from build123d import *

# Parameters (mm, degrees)
SKETCH1_W            = 85.6
SKETCH1_H            = 56
BOSS_EXTRUDE1_DEPTH  = 1.6
SKETCH2_W            = 21.3
SKETCH2_H            = 15.9
BOSS_EXTRUDE2_DEPTH  = 13.5
SKETCH3_W            = 17.4
SKETCH3_H            = 14.7
BOSS_EXTRUDE3_DEPTH  = 15.5
SKETCH4_W            = 16.8
SKETCH4_H            = 28.8
BOSS_EXTRUDE4_DEPTH  = 3.4
SKETCH5_W            = 24
SKETCH5_H            = 2.1
BOSS_EXTRUDE5_DEPTH  = 17.7
SKETCH6_W            = 10
SKETCH6_H            = 10
BOSS_EXTRUDE6_DEPTH  = 13.2
SKETCH7_R            = 4.15
BOSS_EXTRUDE7_DEPTH  = 9.5
SKETCH8_W            = 12
SKETCH8_H            = 11.5
BOSS_EXTRUDE8_DEPTH  = 10
SKETCH9_R            = 3.5
BOSS_EXTRUDE9_DEPTH  = 3.5
SKETCH10_W           = 33
SKETCH10_H           = 5.1
BOSS_EXTRUDE10_DEPTH = 8.3
SKETCH11_W           = 5.4
SKETCH11_H           = 7.5
BOSS_EXTRUDE11_DEPTH = 2.7
SKETCH12_W           = 15
SKETCH12_H           = 9
BOSS_EXTRUDE12_DEPTH = 6.2
SKETCH13_R           = 1.45
CUT_EXTRUDE1_DEPTH   = 6


with BuildPart() as part:
    # Sketch1 → Boss-Extrude1 (new body)
    with BuildSketch(Plane(origin=(0, 0, 0), x_dir=(1, 0, 0), z_dir=(0, 1, 0))):
        Rectangle(SKETCH1_W, SKETCH1_H)
    extrude(amount=BOSS_EXTRUDE1_DEPTH)

    # Sketch2 → Boss-Extrude2 (add)
    with BuildSketch(Plane(origin=(0, 1.6, 0), x_dir=(1, 0, 0), z_dir=(0, 1, 0))):
        with Locations((33.85, -18.45)):
            Rectangle(SKETCH2_W, SKETCH2_H)
    extrude(amount=BOSS_EXTRUDE2_DEPTH)

    # Sketch3 → Boss-Extrude3 (add)
    with BuildSketch(Plane(origin=(0, 1.6, 0), x_dir=(1, 0, 0), z_dir=(0, 1, 0))):
        with Locations((41.7, 2.65)):
            Rectangle(SKETCH3_W, SKETCH3_H)
    extrude(amount=BOSS_EXTRUDE3_DEPTH)

    # Sketch4 → Boss-Extrude4 (add)
    with BuildSketch(Plane.XZ):
        with Locations((-34.4, -1.5)):
            Rectangle(SKETCH4_W, SKETCH4_H)
    extrude(amount=BOSS_EXTRUDE4_DEPTH)

    # Sketch5 → Boss-Extrude5 (add)
    with BuildSketch(Plane.ZY.offset(42.8)):
        with Locations((-2.5, -1.65)):
            Rectangle(SKETCH5_W, SKETCH5_H)
    extrude(amount=BOSS_EXTRUDE5_DEPTH)

    # Sketch6 → Boss-Extrude6 (add)
    with BuildSketch(Plane(origin=(0, 1.6, 0), x_dir=(1, 0, 0), z_dir=(0, 1, 0))):
        with Locations((3.1, 23)):
            Rectangle(SKETCH6_W, SKETCH6_H)
    extrude(amount=BOSS_EXTRUDE6_DEPTH)

    # Sketch7 → Boss-Extrude7 (add)
    with BuildSketch(Plane(origin=(0, 0, -28), x_dir=(-1, 0, 0), z_dir=(0, 0, -1))):
        with Locations((-3.1, 9.4)):
            Circle(SKETCH7_R)
    extrude(amount=BOSS_EXTRUDE7_DEPTH)

    # Sketch8 → Boss-Extrude8 (add)
    with BuildSketch(Plane(origin=(0, 1.6, 0), x_dir=(1, 0, 0), z_dir=(0, 1, 0))):
        with Locations((22.5, 22.25)):
            Rectangle(SKETCH8_W, SKETCH8_H)
    extrude(amount=BOSS_EXTRUDE8_DEPTH)

    # Sketch9 → Boss-Extrude9 (add)
    with BuildSketch(Plane(origin=(0, 0, -28), x_dir=(-1, 0, 0), z_dir=(0, 0, -1))):
        with Locations((-22.5, 8.1)):
            Circle(SKETCH9_R)
    extrude(amount=BOSS_EXTRUDE9_DEPTH)

    # Sketch10 → Boss-Extrude10 (add)
    with BuildSketch(Plane(origin=(0, 1.6, 0), x_dir=(1, 0, 0), z_dir=(0, 1, 0))):
        with Locations((-25.6, 24.55)):
            Rectangle(SKETCH10_W, SKETCH10_H)
    extrude(amount=BOSS_EXTRUDE10_DEPTH)

    # Sketch11 → Boss-Extrude11 (add)
    with BuildSketch(Plane(origin=(0, 1.6, 0), x_dir=(1, 0, 0), z_dir=(0, 1, 0))):
        with Locations((-40.1, -20.75)):
            Rectangle(SKETCH11_W, SKETCH11_H)
    extrude(amount=BOSS_EXTRUDE11_DEPTH)

    # Sketch12 → Boss-Extrude12 (add)
    with BuildSketch(Plane(origin=(0, 1.6, 0), x_dir=(1, 0, 0), z_dir=(0, 1, 0))):
        with Locations((2.5, -23.5)):
            Rectangle(SKETCH12_W, SKETCH12_H)
    extrude(amount=BOSS_EXTRUDE12_DEPTH)

    # Sketch13 → Cut-Extrude1 (cut, through all)
    with BuildSketch(Plane(origin=(0, 1.6, 0), x_dir=(1, 0, 0), z_dir=(0, 1, 0))):
        with Locations((-17.3, -10)):
            Circle(SKETCH13_R)
        with Locations((37.8, 15.5)):
            Circle(SKETCH13_R)
    extrude(amount=-CUT_EXTRUDE1_DEPTH, mode=Mode.SUBTRACT)


solid = part.part
Source: CAD feature listing. Evaluate the final solid. Frame: model axes, mm. A direction names the side the tool comes from. Coordinates: 2 decimals unless noted, no trailing zeros. Order: outer loops, then holes, each group sorted by start corner. A loop starts at its lowest first (then second) coordinate and runs counter-clockwise, first axis right, second up. Notation, with made-up numbers: M 89.25,-16.5 L 111.25,-16.5 A22 cw 111.25,18.5 Z; hole C 29,33 d9. An arc over 180 degrees is marked long. Write each question's results on one line, items separated by ' | '. Start each with the question number.
Item 1: Cut plane A-A (x = 3.1). Return loops of the section in (y, z).
Item 2: Cut plane B-B (z = 1.5). Return loops of the section in (x, y), and give its area (3 significant figures).
Item 3: Line query: probe 1 along X at (y, z) = (0.5, 10); probe 2 along Z at (x, y) = (-0.5, 7.5); probe 3 along Z at (x, y) = (37.8, 1.2). Output: solid intervals per line, ascending.
Item 4: First-contact query: pin 1 Ø1.5 at (y, z) = (5, -23.5) entering from -X; pin 2 Ø7 at (x, y) = (35, 10) entering from -Z; pin 3 Ø3 at (x, y) = (-39.5, 3.5) entering from -Z; pin 4 Ø6 at (x, y) = (-40.5, 14) entering from +Z (3 decimals). Flat tips, straight axial feed; report the tip coordinate or a pass-through.
Item 5: Set-up query: faces 1 (the face through (-52, -2, -14.5)), 2 (the face through (-26, 9.9, -25)), 3 (the face through (2, 7.8, 23)), 4 (the face through (-35, -2, 12.9)). Return all of +Z, -Z, +X, -X, +Y, -Y with unobstructed straight access to the full face (end or side cutting, diameter ignored); none if empty.
Item 6: Draft query along X for faces 5 (the face through (23, 8, -31.5)), 6 (the face through (-60.5, -2, -3)), 7 (the face through (-9.1, 6, -25)). Return one class per face: pulls with the +X half, pulls with the -X half, needs draft (parallel to the pull), parting line crosses it, or undercut.
Item 7: Cut plane C-C (x = -32.5). Return loops of the section in (y, z), and give its area (3 significant figures).
Checked values:
1) outline: M 0,-28 L 5.25,-28 L 5.25,-37.5 L 13.55,-37.5 L 13.55,-28 L 14.8,-28 L 14.8,-18 L 1.6,-18 L 1.6,19 L 7.8,19 L 7.8,28 L 0,28 Z
2) outline: M -60.5,-2.7 L -42.8,-2.7 L -42.8,-3.4 L -26,-3.4 L -26,0 L 42.8,0 L 42.8,1.6 L 50.4,1.6 L 50.4,17.1 L 33,17.1 L 33,1.6 L -42.8,1.6 L -42.8,-0.6 L -60.5,-0.6 Z | area: 501 mm2
3) probe 1: x = -42.8 to -18.75, -15.85 to 42.8 | probe 2: z = -37.5 to -18, 19 to 28 | probe 3: z = -28 to -16.95, -14.05 to 28
4) pin 1: stops at x = -42.1 | pin 2: stops at z = -10 | pin 3: stops at z = -27.1 | pin 4: passes through
5) face 1: -Z, -X, +Y, -Y | face 2: +Z, -Z, -X, +Y | face 3: +Z, -X, +Y | face 4: +Z, +X, -X, -Y
6) face 5: needs draft | face 6: pulls with the -X half | face 7: undercut
7) outline: M -3.4,-15.9 L 0,-15.9 L 0,-28 L 1.6,-28 L 1.6,-27.1 L 9.9,-27.1 L 9.9,-22 L 1.6,-22 L 1.6,28 L 0,28 L 0,12.9 L -3.4,12.9 Z | area: 230 mm2
